Job drawing, mm, ordinate dimensions from the low corner. One solid piece. Coordinates: 2 decimals unless noted, no trailing zeros. Loops run counter-clockwise (first coordinate to the right, second up) from the corner with the lowest first, then second, coordinate; pieces in that order, holes last. Notation, with made-up numbers: (70.25, -37) - (129.25, -37) arc R17 cw to (129.25, -22) - close; hole circle Ø8 at (57.25, -27). An arc over 180 degrees is marked (long way). Use a Markdown table: item, result. Add a question column.
1. Band-saw the part on B-B, the plane y = 3.55. Count the separate pieces of the cut face and the enclosed holes in it, plus the area to 3 significant figures.
2. Band-saw the part on A-A, the plane x = 192.5. Give the cut face in (y, z), plus the area to 3 significant figures.
3. Wall check: probe 1 along X at (y, z) = (2.2, 235); probe 2 along Z at (x, y) = (39.5, 4.3) (1 decimal); probe 3 along Z at (x, y) = (182.5, 2.25). Give the ranges that are in metal, low to high. Write a range as [from, to].
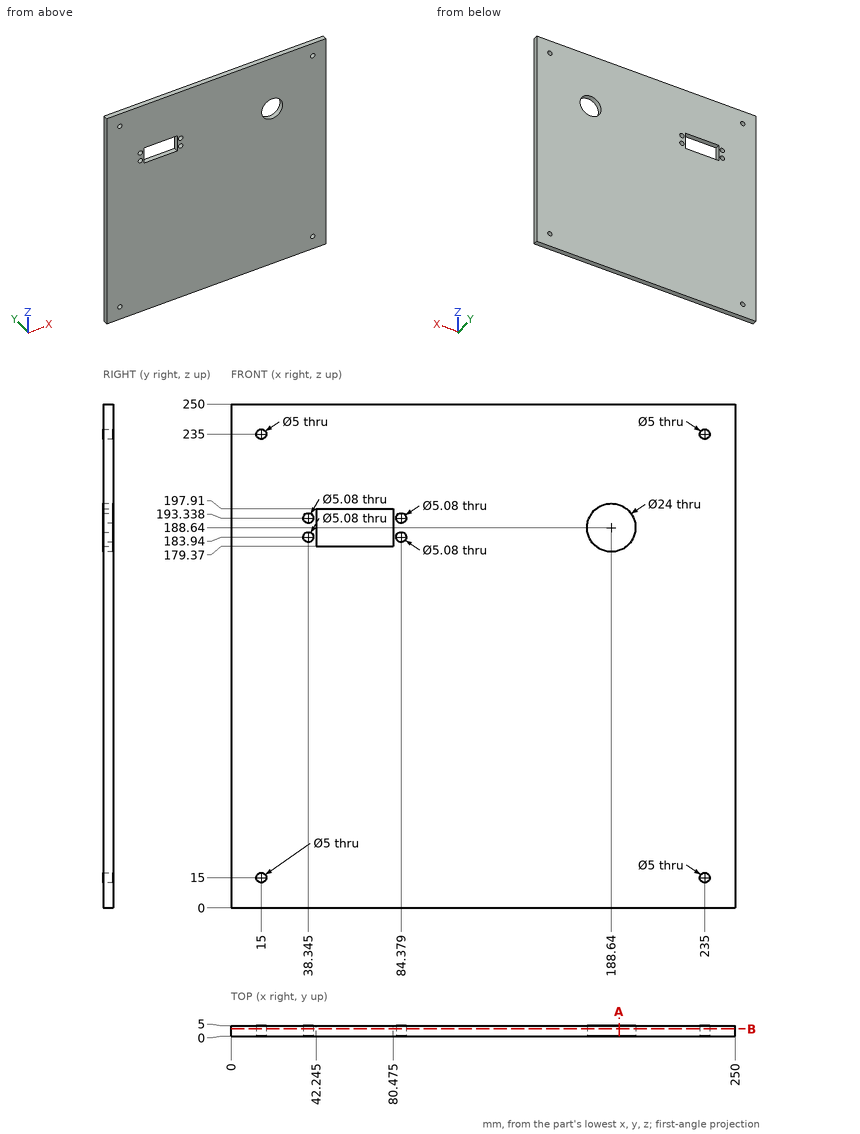
Geometry check:
| question | item | result |
|---|---|---|
| 1 | separate pieces | 1 |
| 1 | enclosed holes | 10 |
| 1 | area | 61,200 mm^2 |
| 2 | outline | (0, 0) - (5, 0) - (5, 177.28) - (0, 177.28) - close; (0, 200) - (5, 200) - (5, 250) - (0, 250) - close |
| 2 | area | 1,140 mm^2 |
| 3 | probe 1 | x = [0, 12.5], [17.5, 232.5], [237.5, 250] |
| 3 | probe 2 | z = [0, 181.7], [186.2, 191.1], [195.6, 250] |
| 3 | probe 3 | z = [0, 178.33], [198.95, 250] |
